The listing builds one solid part. Answer for the finished solid, in the listing's coordinates (mm). Give positions to 0.01 mm unless a question says otherwise; leave off trailing zeros. Write each loop counter-clockwise with the first axis right and the second up, starting at its lowest first coordinate (ties: lowest second). Pieces come first, ordered by that corner, then holes. Notation, with made-up numbers: M -21,-11 L 13,-11 A10 ccw 13,7 Z; hole C 18,-23 d1. An arc over 180 degrees is marked long. Answer as a JSON object with one key per item and string values.
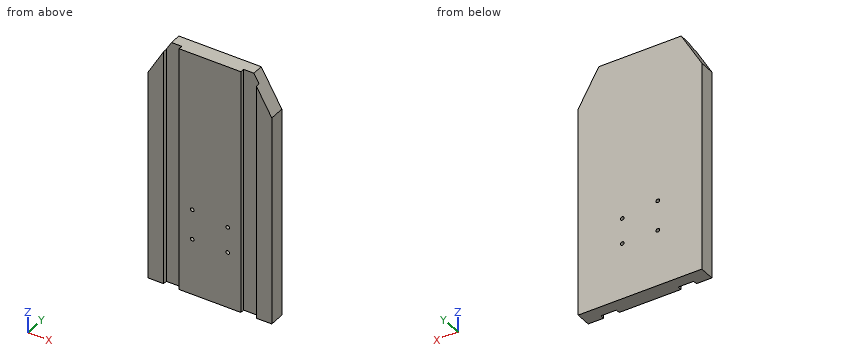
```python
from build123d import *

# Parameters (mm, degrees)
SKETCH1_W             = 152.4
SKETCH1_H             = 304.8
BOSS_EXTRUDE1_DEPTH   = 19.05
F_8_CLEARANCE_HOLE1_D = 4.4958
CUT_EXTRUDE1_DEPTH    = 20.05
SKETCH5_W             = 19.05
SKETCH5_H             = 304.8
CUT_EXTRUDE2_DEPTH    = 5.08


with BuildPart() as part:
    # Sketch1 → Boss-Extrude1 (new body)
    with BuildSketch(Plane(origin=(0, 0, 0), x_dir=(1, 0, 0), z_dir=(0, 1, 0))):
        Rectangle(SKETCH1_W, SKETCH1_H)
    extrude(amount=BOSS_EXTRUDE1_DEPTH)

    # #8 Clearance Hole1 (through all)
    with Locations(Plane(origin=(0, 19.05, 0), x_dir=(1, 0, 0), z_dir=(0, 1, 0))):
        with Locations((-21.89, 82.55), (21.89, 82.55), (-21.89, 45.212), (21.89, 50.8)):
            Hole(F_8_CLEARANCE_HOLE1_D / 2)

    # Sketch4 → Cut-Extrude1 (cut, through all)
    with BuildSketch(Plane.XZ):
        Polygon((76.2, 152.4), (50.8, 152.4), (76.2, 108.405909488), align=None)
        Polygon((-76.2, 108.405909488), (-50.8, 152.4), (-76.2, 152.4), align=None)
    extrude(amount=-CUT_EXTRUDE1_DEPTH, mode=Mode.SUBTRACT)

    # Sketch5 → Cut-Extrude2 (cut)
    with BuildSketch(Plane.XZ):
        with Locations((47.625, 0)):
            Rectangle(SKETCH5_W, SKETCH5_H)
        with Locations((-47.625, 0)):
            Rectangle(SKETCH5_W, SKETCH5_H)
    extrude(amount=-CUT_EXTRUDE2_DEPTH, mode=Mode.SUBTRACT)


solid = part.part
```
1. A cutting plane is placed at D-D, the plane z = 128. Give the vertices of the cut face in (x, y).
Verdict:
{"outline": "M -64.89,0 L -57.15,0 L -57.15,5.08 L -38.1,5.08 L -38.1,0 L 38.1,0 L 38.1,5.08 L 57.15,5.08 L 57.15,0 L 64.89,0 L 64.89,19.05 L -64.89,19.05 Z"}
2. A cutting plane is placed at C-C, the plane x = 63. Give the vertices of the cut face in (y, z).
Verdict:
{"outline": "M 0,-152.4 L 19.05,-152.4 L 19.05,131.27 L 0,131.27 Z"}
3. Consider line 1 along Z through (x, y) = (-21.89, 12); line 2 along X through (y, z) = (3.25, 10); line 3 along Z through (x, y) = (21.89, 13.5). Determine where each line is inside the solid, lowest interval first.
Verdict:
{"line 1": "z = -152.4 to -84.8, -80.3 to -47.46, -42.96 to 152.4", "line 2": "x = -76.2 to -57.15, -38.1 to 38.1, 57.15 to 76.2", "line 3": "z = -152.4 to -84.8, -80.3 to -53.05, -48.55 to 152.4"}
4. A cutting plane is placed at A-A, the plane z = -124. Give the vertices of the cut face in (x, y), plus the area to 3 significant figures.
Verdict:
{"outline": "M -76.2,0 L -57.15,0 L -57.15,5.08 L -38.1,5.08 L -38.1,0 L 38.1,0 L 38.1,5.08 L 57.15,5.08 L 57.15,0 L 76.2,0 L 76.2,19.05 L -76.2,19.05 Z", "area": "2,710 mm2"}
5. Flat-ended cylindrical pins translate along their axes: pin 1 (4 mm diameter, centred on x = -21.89, z = -82.55, fed in from -Y); pin 2 (5.5 mm diameter, centred on x = -50, z = -31.5, fed in from -Y). Find the tip coordinate at first contact, or state that the pin passes through.
Verdict:
{"pin 1": "passes through", "pin 2": "stops at y = 5.08"}
6. A cutting plane is placed at B-B, the plane y = 16.25. Give the vertices of the cut face in (x, z).
Verdict:
{"outline": "M -76.2,-152.4 L 76.2,-152.4 L 76.2,108.41 L 50.8,152.4 L -50.8,152.4 L -76.2,108.41 Z; hole C -21.89,-82.55 d4.5; hole C -21.89,-45.21 d4.5; hole C 21.89,-82.55 d4.5; hole C 21.89,-50.8 d4.5"}
